Design review of the part shown in the three views and the two pictorial views. Dimensions are in mm from the part's minimum x, y and z. A direction names the side the tool comes from. Give positions to 0.01 mm unless a question says otherwise; leave off trailing zeros. Loops run counter-clockwise (first coordinate to the right, second up) from the corner with the lowest first, then second, coordinate; pieces in that order, holes last. Notation, with made-up numbers: (20.5, -20.75) -> (56.5, -20.75) arc R32 ccw to (56.5, 16.25) -> close; hole circle Ø7 at (40.5, 60). An arc over 180 degrees is marked (long way). One line per question, with ' | ' between items. Start each with the question number.
(1) Consider section C-C (z = 6.75). Write out the cut boundary in (x, y).
(2) Consider section B-B (y = 31.75). Write out the cut boundary in (x, z).
(3) Insertion check: P1, Ø4, axis at x = 12.7, y = 6.35, coming from the +Z side. The pin has a flat end and moves straight along its axis. Give the tip position at first contact, or say it passes through.
(4) Draft analysis for pull direction Z (two halves, no side actions). For the marked faces 1, 2, 3 and 4, state which applies: +Z half, -Z half, draft (parallel to the pull), parting line (faces both ways), or undercut.
(5) Tool access review of the marked faces 5 and 6: name each direction out of +Z, -Z, +X, -X, +Y, -Y from which nothing blocks a thin tool from reaching the whole face with its end or side.
(6) Wall thickness on probe 1 along Y at (x, z) = (12.7, 24.7); probe 2 along Z at (x, y) = (16.75, 13): over which ranges is each line inside the solid? List them lowest first.
(7) Consider section D-D (x = 4). Write out the cut boundary in (y, z).
(8) Consider section A-A (x = 12.7). Give the number of separate pieces and of enclosed holes in the cut face, and give its area (3 significant figures).
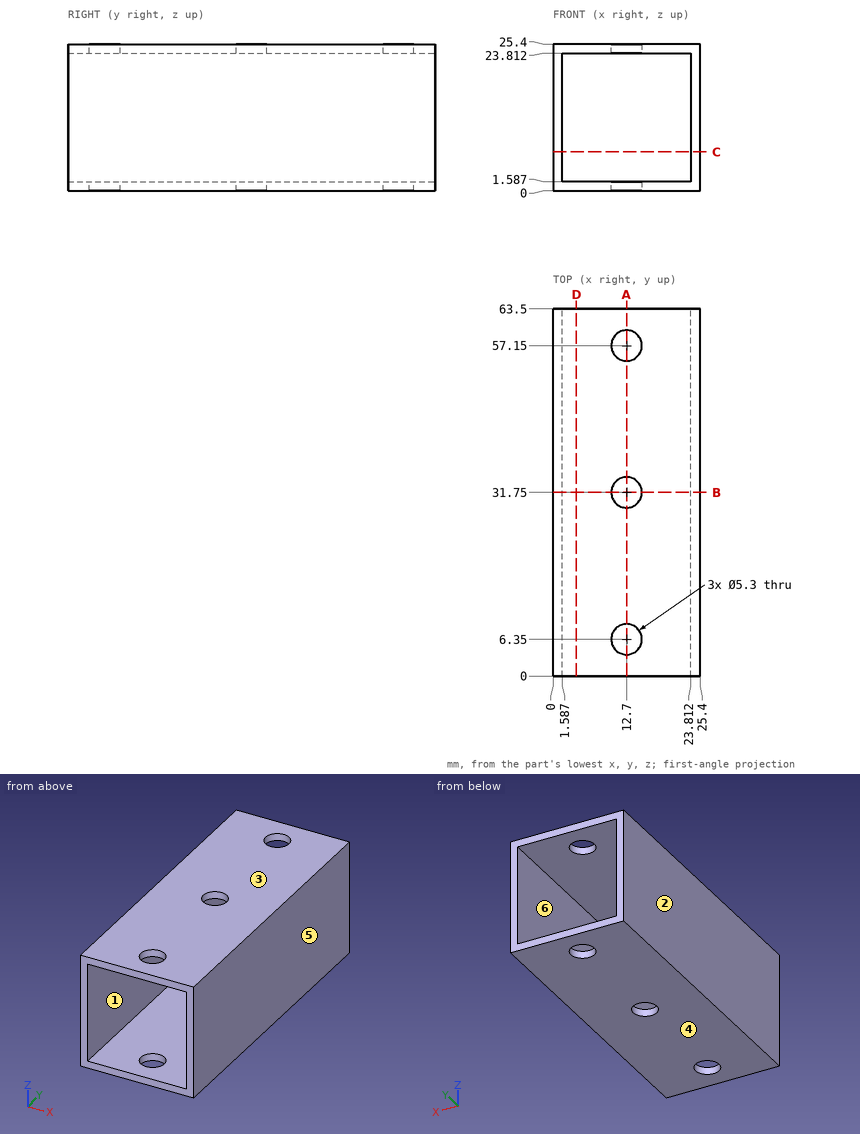
A:
1) outline: (0, 0) -> (1.59, 0) -> (1.59, 63.5) -> (0, 63.5) -> close; (23.81, 0) -> (25.4, 0) -> (25.4, 63.5) -> (23.81, 63.5) -> close
2) outline: (0, 0) -> (10.05, 0) -> (10.05, 1.59) -> (1.59, 1.59) -> (1.59, 23.81) -> (10.05, 23.81) -> (10.05, 25.4) -> (0, 25.4) -> close; (15.35, 0) -> (25.4, 0) -> (25.4, 25.4) -> (15.35, 25.4) -> (15.35, 23.81) -> (23.81, 23.81) -> (23.81, 1.59) -> (15.35, 1.59) -> close
3) P1: passes through
4) face 1: undercut | face 2: draft | face 3: +Z half | face 4: -Z half
5) face 5: +Z, -Z, +X, +Y, -Y | face 6: +Y, -Y
6) probe 1: y = 0 to 3.7, 9 to 29.1, 34.4 to 54.5, 59.8 to 63.5 | probe 2: z = 0 to 1.59, 23.81 to 25.4
7) outline: (0, 0) -> (63.5, 0) -> (63.5, 1.59) -> (0, 1.59) -> close; (0, 23.81) -> (63.5, 23.81) -> (63.5, 25.4) -> (0, 25.4) -> close
8) separate pieces: 8 | enclosed holes: 0 | area: 151 mm^2
